from build123d import *

# Parameters (mm, degrees)
SKETCH2_W          = 1.42
SKETCH2_H          = 2.59
SKETCH2_W_2        = 2.59
SKETCH2_H_2        = 1.42
CUT_EXTRUDE1_DEPTH = 2.64
DRAFT1_ANGLE       = 26.5
CHAMFER1_SIZE      = 0.5


with BuildPart() as part:
    # Sketch1 → Revolve1 (revolve)
    with BuildSketch(Plane.XY):
        Polygon((0, 0), (0, 5.65), (-0.65, 5.65), (-3.3, 3), (-20, 3), (-20, 0), align=None)
    revolve(axis=Axis((0, 0, 0), (-1, 0, 0)))

    # Sketch2 → Cut-Extrude1 (cut)
    with BuildSketch(Plane(origin=(0, 0, 0), x_dir=(0, 0, -1), z_dir=(1, 0, 0))):
        with Locations((0, 2.005)):
            Rectangle(SKETCH2_W, SKETCH2_H)
        with Locations((-2.005, 0)):
            Rectangle(SKETCH2_W_2, SKETCH2_H_2)
        Rectangle(SKETCH2_W, SKETCH2_H_2)
        with Locations((2.005, 0)):
            Rectangle(SKETCH2_W_2, SKETCH2_H_2)
        with Locations((0, -2.005)):
            Rectangle(SKETCH2_W, SKETCH2_H)
    extrude(amount=-CUT_EXTRUDE1_DEPTH, mode=Mode.SUBTRACT)

    # Draft1
    draft1_faces = [part.faces().sort_by_distance(p)[0] for p in [
        (-1.32, 0, -3.3),
        (-1.32, -3.3, 0),
        (-1.32, 0, 3.3),
        (-1.32, 3.3, 0),
    ]]
    draft(draft1_faces, Plane.YZ, DRAFT1_ANGLE)

    # Chamfer1
    chamfer1_edges = [part.edges().sort_by_distance(p)[0] for p in [
        (-20, -3, 0),
    ]]
    chamfer(chamfer1_edges, length=CHAMFER1_SIZE)


solid = part.part
Read the model definition and answer for the solid it produces. Units are mm, in the model's axes. A direction names the side the tool comes from. Give positions to 0.01 mm unless a question says otherwise; leave off trailing zeros. Write each loop counter-clockwise with the first axis right and the second up, starting at its lowest first coordinate (ties: lowest second). Pieces come first, ordered by that corner, then holes. Notation, with made-up numbers: (50.25, 84) - (55.25, 84) arc R26 cw to (55.25, 117) - close; hole circle Ø11 at (-16.75, 17). An arc over 180 degrees is marked (long way). Return JSON: item names as keys, results as strings.
Q1. Consider line 1 along Y through (x, z) = (-1.5, 1.75); line 2 along X through (y, z) = (-0.75, -4.25); line 3 along Z through (x, y) = (-1.5, 2). Determine where each line is inside the solid, lowest interval first. Write a range as [from, to].
Reply:
{"line 1": "[-4.47, -0.71], [0.71, 4.47]", "line 2": "[-1.98, 0]", "line 3": "[-4.36, -0.71], [0.71, 4.36]"}
Q2. For a pull along Z with two mould halves and no side action, classify faces 3 (the face through (-1.3, 2.65, 0.01)), 4 (the face through (-20, 0, 0)), 5 (the face through (-1, 2, 0.71)), 6 (the face through (-12, -3, 0)) as released by +Z, released by -Z, zero draft, split by the parting line, or undercut.
Reply:
{"face 3": "undercut", "face 4": "zero draft", "face 5": "undercut", "face 6": "split by the parting line"}
Q3. Given P1, Ø1.3, axis at x = -1.5, y = 2.5, coming from the -Z side; P2, Ø0.8, axis at x = -1.5, z = -2.5, coming from the -Y side; P3, Ø2, axis at x = -2, y = -2.5, coming from the -Z side, each flat-ended and moving along its own axis, determine where each tip first touches the part or whether it passes through.
Reply:
{"P1": "z = -4.91", "P2": "y = -4.61", "P3": "z = -4.78"}
Q4. A cutting plane is placed at A-A, the plane z = 0. Determine the outline of the cut face in (x, y), and give its area (3 significant figures).
Reply:
{"outline": "(-20, -2.5) - (-19.5, -3) - (-3.3, -3) - (-0.65, -5.65) - (0, -5.65) - (0, -3.3) - (-2.64, -1.98) - (-2.64, 1.98) - (0, 3.3) - (0, 5.65) - (-0.65, 5.65) - (-3.3, 3) - (-19.5, 3) - (-20, 2.5) - close", "area": "116 mm²"}
Q5. A cutting plane is placed at C-C, the plane x = -3. Determine the outline of the cut face in (y, z).
Reply:
{"outline": "circle Ø6.6 at (0, 0)"}
Q6. For faces 1 (the face through (-0.33, 5.39, -1.7)), 2 (the face through (-1.3, -2.65, 0.01)), determine the directions among +Z, -Z, +X, -X, +Y, -Y from which every point of the face is accessible in a straight line to the end or side of a thin tool.
Reply:
{"face 1": "+X, -X", "face 2": "+X"}
